```python
from build123d import *

# Parameters (mm, degrees)
F0_R     = 25
F1_DEPTH = 25
F2_R     = 15
F3_DEPTH = 50
F4_R     = 0.5


with BuildPart() as f1:
    # F0 (on Right) → F1 (new body, symmetric)
    with BuildSketch(Plane.YZ):
        Circle(F0_R)
    extrude(amount=F1_DEPTH, both=True)

    # F2 (on Top) → F3 (join)
    with BuildSketch(Plane.XY):
        Circle(F2_R)
    extrude(amount=-F3_DEPTH)

    # F4
    f4_edges = [f1.edges().sort_by_distance(p)[0] for p in [
        (-15, 0, -25),
    ]]
    fillet(f4_edges, radius=F4_R)


solid = f1.part
```
Verification items for the finished model (mm, model axes). Coordinates: 2 decimals unless noted, no trailing zeros. Order: outer loops, then holes, each group sorted by start corner. A loop starts at its lowest first (then second) coordinate and runs counter-clockwise, first axis right, second up. Notation, with made-up numbers: (81.5, -18.5) -> (92.5, -18.5) arc R18 ccw to (92.5, -11.5) -> close; hole circle Ø8 at (57.5, -8). An arc over 180 degrees is marked (long way). Put each result on its own line as item: value. Start each with the question number.
1) Cross-section at A-A (z = -36). Enter the section's corners in (x, y), plus the area to 3 significant figures.
2) Cross-section at C-C (z = 18). Enter the section's corners in (x, y), plus the area to 3 significant figures.
3) Release check for a two-part mould opening along X. For faces 1 (the flat face through (0, 0, -50)), 2 (the flat face through (-25, 0, 0)), 3 (the cylindrical face through (-3.252, -14.643, -34.915)) record: pulls with the +X half, pulls with the -X half, needs draft (parallel to the pull), parting line crosses it, or undercut.
4) Go/stop test with flat-tipped pins: pin 1 (12 mm diameter, centred on x = 18.5, z = 8.5, fed in from +Y); pin 2 (3 mm diameter, centred on x = -9, y = -5.5, fed in from +Z); pin 3 (2 mm diameter, centred on x = 4, z = 10.5, fed in from +Y). Record where each tip stops, or that it passes through.
5) Cross-section at B-B (y = 20.5). Enter the section's corners in (x, z).
6) Material ranges on L1, parallel to Z at x = 8, y = 0.5 (3 decimals); L2, parallel to Z at x = -2, y = 10; L3, parallel to Y at x = 20.5, z = -6.5, recorded low to high.
Geometry check:
1. outline: circle Ø30 at (0, 0)
1. area: 707 mm^2
2. outline: (-25, -17.35) -> (25, -17.35) -> (25, 17.35) -> (-25, 17.35) -> close
2. area: 1,730 mm^2
3. face 1: needs draft
3. face 2: pulls with the -X half
3. face 3: parting line crosses it
4. pin 1: stops at y = 24.87
4. pin 2: stops at z = 24.68
4. pin 3: stops at y = 23.12
5. outline: (-25, -14.31) -> (25, -14.31) -> (25, 14.31) -> (-25, 14.31) -> close
6. L1: z = -50 to 24.995
6. L2: z = -50 to 22.91
6. L3: y = -24.14 to 24.14
